Check sheet for the modelled part. Datum: model origin and axes. Units: mm. Face numbers are marked on the shaded views. A direction names the side the tool comes from. Give positions to 0.01 mm unless a question says otherwise; leave off trailing zeros. Order: outer loops, then holes, each group sorted by start corner. A loop starts at its lowest first (then second) coordinate and runs counter-clockwise, first axis right, second up. Notation, with made-up numbers: (76, -39.5) -> (86, -39.5) arc R19 cw to (86, -8.5) -> close; hole circle Ø1 at (69.5, -31). An arc over 180 degrees is marked (long way). Write each question's results on one line, items separated by ' | '.
from build123d import *

# Parameters (mm, degrees)
SKETCH1_W           = 5
SKETCH1_H           = 8.7
BOSS_EXTRUDE2_DEPTH = 2
SKETCH2_R           = 1.5
CUT_EXTRUDE1_DEPTH  = 1
SKETCH3_R           = 0.6
CUT_EXTRUDE2_DEPTH  = 1
SKETCH4_W           = 5
SKETCH4_H           = 2
BOSS_EXTRUDE4_DEPTH = 15
SKETCH6_R           = 1.25
CUT_EXTRUDE4_DEPTH  = 2
CHAMFER1_SIZE       = 1


with BuildPart() as part:
    # Sketch1 → Boss-Extrude2 (new body)
    with BuildSketch(Plane.XY):
        with Locations((0, -1.85)):
            Rectangle(SKETCH1_W, SKETCH1_H)
    extrude(amount=BOSS_EXTRUDE2_DEPTH)

    # Sketch2 → Cut-Extrude1 (cut)
    with BuildSketch(Plane.XY.offset(2)):
        Circle(SKETCH2_R)
    extrude(amount=-CUT_EXTRUDE1_DEPTH, mode=Mode.SUBTRACT)

    # Sketch3 → Cut-Extrude2 (cut)
    with BuildSketch(Plane.XY.offset(1)):
        Circle(SKETCH3_R)
    extrude(amount=-CUT_EXTRUDE2_DEPTH, mode=Mode.SUBTRACT)

    # Sketch4 → Boss-Extrude4 (add)
    with BuildSketch(Plane(origin=(0, 0, 0), x_dir=(-1, 0, 0), z_dir=(0, 0, -1))):
        with Locations((0, -5.2)):
            Rectangle(SKETCH4_W, SKETCH4_H)
    extrude(amount=BOSS_EXTRUDE4_DEPTH)

    # Sketch6 → Cut-Extrude4 (cut)
    with BuildSketch(Plane(origin=(0, -4.2, 0), x_dir=(1, 0, 0), z_dir=(0, 1, 0))):
        with Locations((0, 10)):
            Circle(SKETCH6_R)
        with Locations((0, 5)):
            Circle(SKETCH6_R)
    extrude(amount=-CUT_EXTRUDE4_DEPTH, mode=Mode.SUBTRACT)

    # Chamfer1
    chamfer1_edges = [part.edges().sort_by_distance(p)[0] for p in [
        (-1.25, -4.2, -10),
        (-1.25, -4.2, -5),
    ]]
    chamfer(chamfer1_edges, length=CHAMFER1_SIZE)


solid = part.part
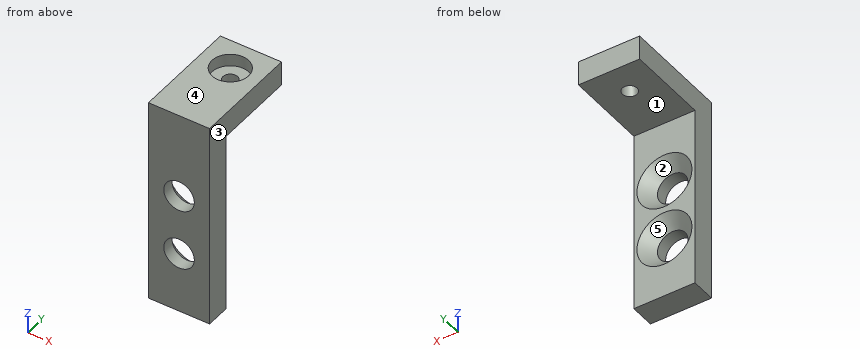
1. Access from +Z, -Z, +X, -X, +Y, -Y to the whole of each face (thin tool, end or side, straight path). Record for the marked faces 1 and 2.
Verdict:
face 1: -Z, +X, -X, +Y | face 2: +Y
2. Gauge pin test, flat ends, axial feed: pin 1 Ø3 at (x, y) = (-1, -2) entering from -Z; pin 2 Ø5 at (y, z) = (1, -4) entering from +X; pin 3 Ø1.5 at (x, z) = (1, -8.5) entering from +Y; pin 4 Ø3 at (x, z) = (0, -10) entering from +Y. Record the tip position at first contact, or that the pin passes through.
Verdict:
pin 1: stops at z = 0 | pin 2: passes through | pin 3: stops at y = -4.2 | pin 4: stops at y = -4.95
3. Section check B-B on y = 0. Record the cut outline in (x, z).
Verdict:
outline: (-2.5, 0) -> (-0.6, 0) -> (-0.6, 1) -> (-1.5, 1) -> (-1.5, 2) -> (-2.5, 2) -> close; (0.6, 0) -> (2.5, 0) -> (2.5, 2) -> (1.5, 2) -> (1.5, 1) -> (0.6, 1) -> close
4. Mould release check, pull along X, two halves, no side actions. Record for the marked faces 3, 4 and 5: +X half, -X half, draft (parallel to the pull), parting line (faces both ways), or undercut.
Verdict:
face 3: +X half | face 4: draft | face 5: undercut
5. Material ranges on probe 1 along Z at (x, y) = (0, -5.45); probe 2 along Y at (x, z) = (0, 1.85); probe 3 along Z at (x, y) = (-0.2, -4.5), recorded low to high. Write a range as from..to.
Verdict:
probe 1: z = -15..-11.25, -8.75..-6.25, -3.75..2 | probe 2: y = -6.2..-1.5, 1.5..2.5 | probe 3: z = -15..-11.94, -8.06..-6.94, -3.06..2
6. Section check A-A on z = -10. Record the cut outline in (x, y), then the cut area to 3 significant figures.
Verdict:
outline: (-2.5, -6.2) -> (-1.25, -6.2) -> (-1.25, -5.2) -> (-2.25, -4.2) -> (-2.5, -4.2) -> close; (1.25, -6.2) -> (2.5, -6.2) -> (2.5, -4.2) -> (2.25, -4.2) -> (1.25, -5.2) -> close | area: 4.00 mm^2
7. Section check D-D on y = -5.5. Record the cut outline in (x, z).
Verdict:
outline: (-2.5, -15) -> (2.5, -15) -> (2.5, 2) -> (-2.5, 2) -> close; hole circle Ø2.5 at (0, -10); hole circle Ø2.5 at (0, -5)
8. Section check C-C on x = 0. Record the cut outline in (y, z), then the cut area to 3 significant figures.
Verdict:
outline: (-6.2, -15) -> (-4.2, -15) -> (-4.2, -12.25) -> (-5.2, -11.25) -> (-6.2, -11.25) -> close; (-6.2, -8.75) -> (-5.2, -8.75) -> (-4.2, -7.75) -> (-4.2, -7.25) -> (-5.2, -6.25) -> (-6.2, -6.25) -> close; (-6.2, -3.75) -> (-5.2, -3.75) -> (-4.2, -2.75) -> (-4.2, 0) -> (-0.6, 0) -> (-0.6, 1) -> (-1.5, 1) -> (-1.5, 2) -> (-6.2, 2) -> close; (0.6, 0) -> (2.5, 0) -> (2.5, 2) -> (1.5, 2) -> (1.5, 1) -> (0.6, 1) -> close | area: 31.2 mm^2
